The figure shows three views and two pictorial views of one solid part (mm, origin at its lowest corner). Answer the questions. Round coordinates to 2 decimals unless told otherwise and drop trailing zeros. Write each loop counter-clockwise with the first axis right and the second up, starting at its lowest first coordinate (ties: lowest second). Pieces come first, ordered by that corner, then holes.
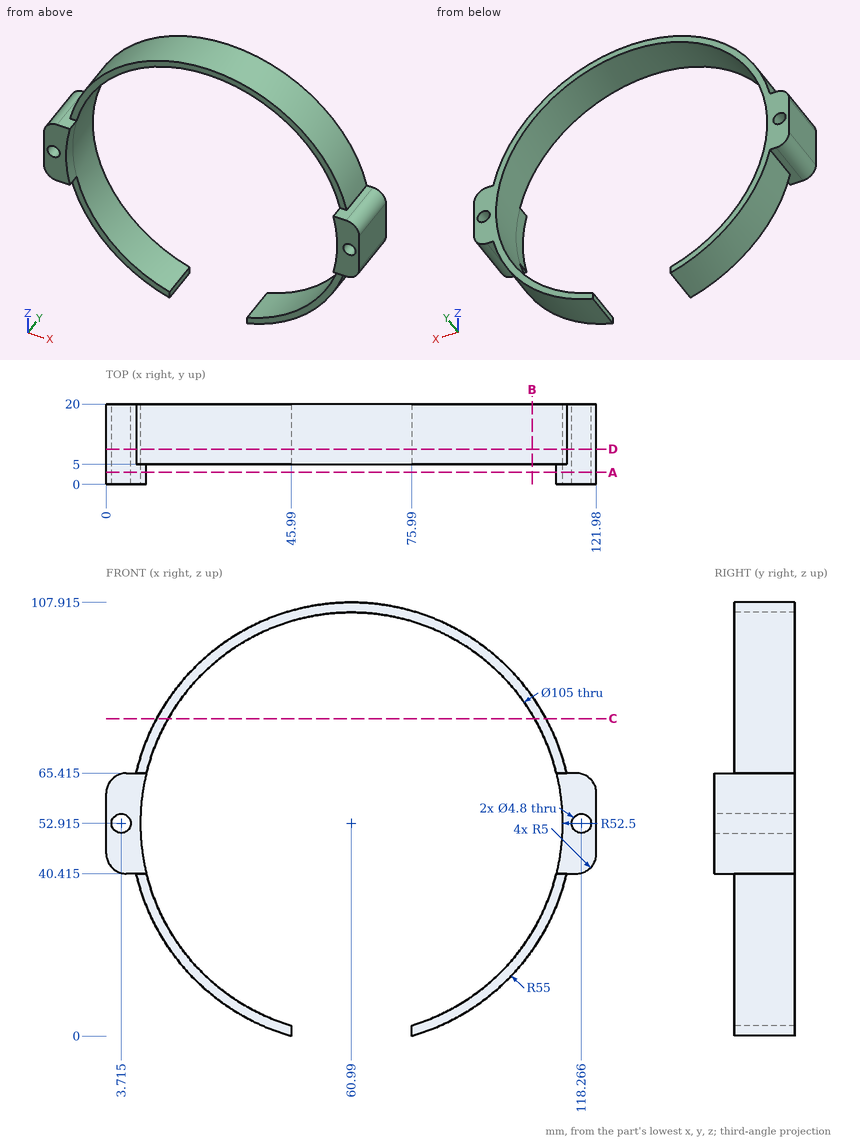
Q1. Flat-ended cylindrical pins translate along their axes: pin 1 Ø5 at (x, y) = (58, 8.5) entering from -Z; pin 2 Ø6 at (x, y) = (19, 10) entering from +Z (1 decimal); pin 3 Ø3 at (y, z) = (14, 1) entering from -X (1 decimal). Find the tip coordinate at first contact, or state that the pin passes through.
Verdict:
pin 1: stops at z = 105.13
pin 2: stops at z = 91.7
pin 3: stops at x = 39
Q2. Section B-B (x = 106) is taken. Determine the outline of the cut face in (y, z).
Verdict:
outline: (5, 21.31) - (20, 21.31) - (20, 25.89) - (5, 25.89) - close; (5, 79.94) - (20, 79.94) - (20, 84.52) - (5, 84.52) - close
Q3. Section C-C (z = 79) is taken. Determine the outline of the cut face in (x, y).
Verdict:
outline: (12.57, 5) - (15.43, 5) - (15.43, 20) - (12.57, 20) - close; (106.55, 5) - (109.41, 5) - (109.41, 20) - (106.55, 20) - close
Q4. Straight lines are drawn through the part: probe 1 along Z at (x, y) = (100.5, 7) (1 decimal); probe 2 along Z at (x, y) = (77.5, 9.75); probe 3 along Z at (x, y) = (60, 9) (1 decimal). For each, find the intervals that lie inside material, in ascending order.
Verdict:
probe 1: z = 14.7 to 18.3, 87.5 to 91.2
probe 2: z = 0.45 to 3.08, 102.75 to 105.38
probe 3: z = 105.4 to 107.9
Q5. Section A-A (y = 3) is taken. Determine the outline of the cut face in (x, z) (1 decimal), then the cut area to 3 significant figures.
Verdict:
outline: (0, 45.4) arc R5 ccw to (5, 40.4) - (10, 40.4) arc R52.5 cw to (10, 65.4) - (5, 65.4) arc R5 ccw to (0, 60.4) - close; (112, 40.4) - (117, 40.4) arc R5 ccw to (122, 45.4) - (122, 60.4) arc R5 ccw to (117, 65.4) - (112, 65.4) arc R52.5 cw to start; hole circle Ø4.8 at (3.7, 52.9); hole circle Ø4.8 at (118.3, 52.9)
area: 392 mm2
Q6. Section D-D (y = 8.75) is taken. Determine the outline of the cut face in (x, z) (1 decimal).
Verdict:
outline: (0, 45.4) arc R5 ccw to (5, 40.4) - (7.4, 40.4) arc R55 ccw to (46, 0) - (46, 2.6) arc R52.5 cw (long way) to (76, 2.6) - (76, 0) arc R55 ccw to (114.6, 40.4) - (117, 40.4) arc R5 ccw to (122, 45.4) - (122, 60.4) arc R5 ccw to (117, 65.4) - (114.6, 65.4) arc R55 ccw to (7.4, 65.4) - (5, 65.4) arc R5 ccw to (0, 60.4) - close; hole circle Ø4.8 at (3.7, 52.9); hole circle Ø4.8 at (118.3, 52.9)
